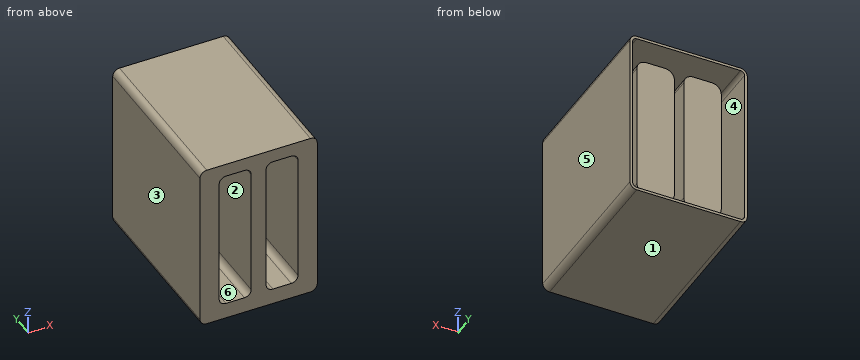
```python
from build123d import *

# Parameters (mm, degrees)
F1_DEPTH = 160
F3_DEPTH = 140
F4_T     = -2.54


with BuildPart() as f1:
    # F0 (on Front) → F1 (new body)
    with BuildSketch(Plane.XZ):
        with BuildLine():
            Line((-103.65, 0), (-6.35, 0))
            ThreePointArc((-6.35, 0), (-1.8598719395, 1.8598719395), (0, 6.35))
            Line((0, 6.35), (0, 153.65))
            ThreePointArc((0, 153.65), (-1.8598719395, 158.1401280605), (-6.35, 160))
            Line((-6.35, 160), (-103.65, 160))
            ThreePointArc((-103.65, 160), (-108.1401280605, 158.1401280605), (-110, 153.65))
            Line((-110, 153.65), (-110, 6.35))
            ThreePointArc((-110, 6.35), (-108.1401280605, 1.8598719395), (-103.65, 0))
        make_face()
    extrude(amount=F1_DEPTH)

    # F2 (on face) → F3 (cut)
    with BuildSketch(Plane.XZ.offset(160)):
        with BuildLine():
            Line((-24.35, 147.7), (-41.65, 147.7))
            ThreePointArc((-41.65, 147.7), (-46.1401280605, 145.8401280605), (-48, 141.35))
            Line((-48, 141.35), (-48, 21.35))
            ThreePointArc((-48, 21.35), (-46.1401280605, 16.8598719395), (-41.65, 15))
            Line((-41.65, 15), (-24.35, 15))
            ThreePointArc((-24.35, 15), (-19.8598719395, 16.8598719395), (-18, 21.35))
            Line((-18, 21.35), (-18, 141.35))
            ThreePointArc((-18, 141.35), (-19.8598719395, 145.8401280605), (-24.35, 147.7))
        make_face()
        with BuildLine():
            Line((-68.35, 147.7), (-85.65, 147.7))
            ThreePointArc((-85.65, 147.7), (-90.1401280605, 145.8401280605), (-92, 141.35))
            Line((-92, 141.35), (-92, 21.35))
            ThreePointArc((-92, 21.35), (-90.1401280605, 16.8598719395), (-85.65, 15))
            Line((-85.65, 15), (-68.35, 15))
            ThreePointArc((-68.35, 15), (-63.8598719395, 16.8598719395), (-62, 21.35))
            Line((-62, 21.35), (-62, 141.35))
            ThreePointArc((-62, 141.35), (-63.8598719395, 145.8401280605), (-68.35, 147.7))
        make_face()
    extrude(amount=-F3_DEPTH, mode=Mode.SUBTRACT)

    # F4
    f4_openings = [f1.faces().sort_by_distance(p)[0] for p in [
        (-55, 0, 80),
    ]]
    offset(amount=F4_T, openings=f4_openings, kind=Kind.INTERSECTION)


solid = f1.part
```
Model file for the job. Use its own axes, mm. Face numbers are marked on the shaded views. A direction names the side the tool comes from. Coordinates: 2 decimals unless noted, no trailing zeros. Order: outer loops, then holes, each group sorted by start corner. A loop starts at its lowest first (then second) coordinate and runs counter-clockwise, first axis right, second up. Notation, with made-up numbers: (85, 1.25) -> (141, 1.25) arc R10 ccw to (141, 9.25) -> close; hole circle Ø5 at (21, 84). An arc over 180 degrees is marked (long way). Return JSON: item names as keys, results as strings.
Item 1: Slice it at B-B (z = 129). Write the cut outline in (x, y).
Model answer:
{"outline": "(-110, -160) -> (-92, -160) -> (-92, -20) -> (-62, -20) -> (-62, -160) -> (-48, -160) -> (-48, -20) -> (-18, -20) -> (-18, -160) -> (0, -160) -> (0, 0) -> (-2.54, 0) -> (-2.54, -157.46) -> (-15.46, -157.46) -> (-15.46, -17.46) -> (-50.54, -17.46) -> (-50.54, -157.46) -> (-59.46, -157.46) -> (-59.46, -17.46) -> (-94.54, -17.46) -> (-94.54, -157.46) -> (-107.46, -157.46) -> (-107.46, 0) -> (-110, 0) -> close"}
Item 2: Slice it at C-C (x = -34). Write the cut outline in (y, z), then the cut area to 3 significant figures.
Model answer:
{"outline": "(-160, 0) -> (0, 0) -> (0, 2.54) -> (-157.46, 2.54) -> (-157.46, 12.46) -> (-17.46, 12.46) -> (-17.46, 150.24) -> (-157.46, 150.24) -> (-157.46, 157.46) -> (0, 157.46) -> (0, 160) -> (-160, 160) -> (-160, 147.7) -> (-20, 147.7) -> (-20, 15) -> (-160, 15) -> close", "area": "1,920 mm²"}
Item 3: Pin check, flat tips, straight feed: P1, Ø6, axis at x = -50.5, z = 86, coming from the +Y side; P2, Ø24, axis at x = -81, z = 64, coming from the -Y side; P3, Ø1, axis at x = -70.5, z = 85.5, coming from the -Y side. Stop position of each tip, or through.
Model answer:
{"P1": "stops at y = -17.46", "P2": "stops at y = -160", "P3": "stops at y = -20"}
Item 4: Wall check: line 1 along Z through (x, y) = (-75.5, -102); line 2 along X through (y, z) = (-105.5, 46.5); line 3 along Z through (x, y) = (-16, -9). Give the ranges that are in metal, low to high. Write a range as from..to.
Model answer:
{"line 1": "z = 0..2.54, 12.46..15, 147.7..150.24, 157.46..160", "line 2": "x = -110..-107.46, -94.54..-92, -62..-59.46, -50.54..-48, -18..-15.46, -2.54..0", "line 3": "z = 0..2.54, 157.46..160"}
Item 5: Slice it at A-A (y = -50). Count the separate pieces of the cut face and the enclosed holes in it, then the cut area to 3 significant figures.
Model answer:
{"separate pieces": "3", "enclosed holes": "3", "area": "2,960 mm²"}
Item 6: Slice it at D-D (x = -10). Write the cut outline in (y, z).
Model answer:
{"outline": "(-160, 0) -> (0, 0) -> (0, 2.54) -> (-157.46, 2.54) -> (-157.46, 157.46) -> (0, 157.46) -> (0, 160) -> (-160, 160) -> close"}
Item 7: Mould opens along X. For the marked faces 1, 2 and 3 say: pulls with the +X half, pulls with the -X half, needs draft (parallel to the pull), parting line crosses it, or undercut.
Model answer:
{"face 1": "needs draft", "face 2": "undercut", "face 3": "pulls with the -X half"}
Item 8: 3-axis set-ups, long thin cutter, end or side, ignore diameter. For the marked faces 4, 5 and 6: which of +Z, -Z, +X, -X, +Y, -Y reach the whole face in a straight line?
Model answer:
{"face 4": "+Y", "face 5": "+Z, -Z, +X, +Y, -Y", "face 6": "-Y"}
